Part print with two shaded views. Sizes in mm from the minimum x, y, z corner. Round coordinates to 2 decimals unless told otherwise and drop trailing zeros. Loops run counter-clockwise (first coordinate to the right, second up) from the corner with the lowest first, then second, coordinate; pieces in that order, holes last. Notation, with made-up numbers: (-40, 76.25) - (-4, 76.25) arc R31 cw to (-4, 107.25) - close; hole circle Ø10 at (-20.5, 75). An arc over 180 degrees is marked (long way). Put each result on its own line as item: value. Start each with the question number.
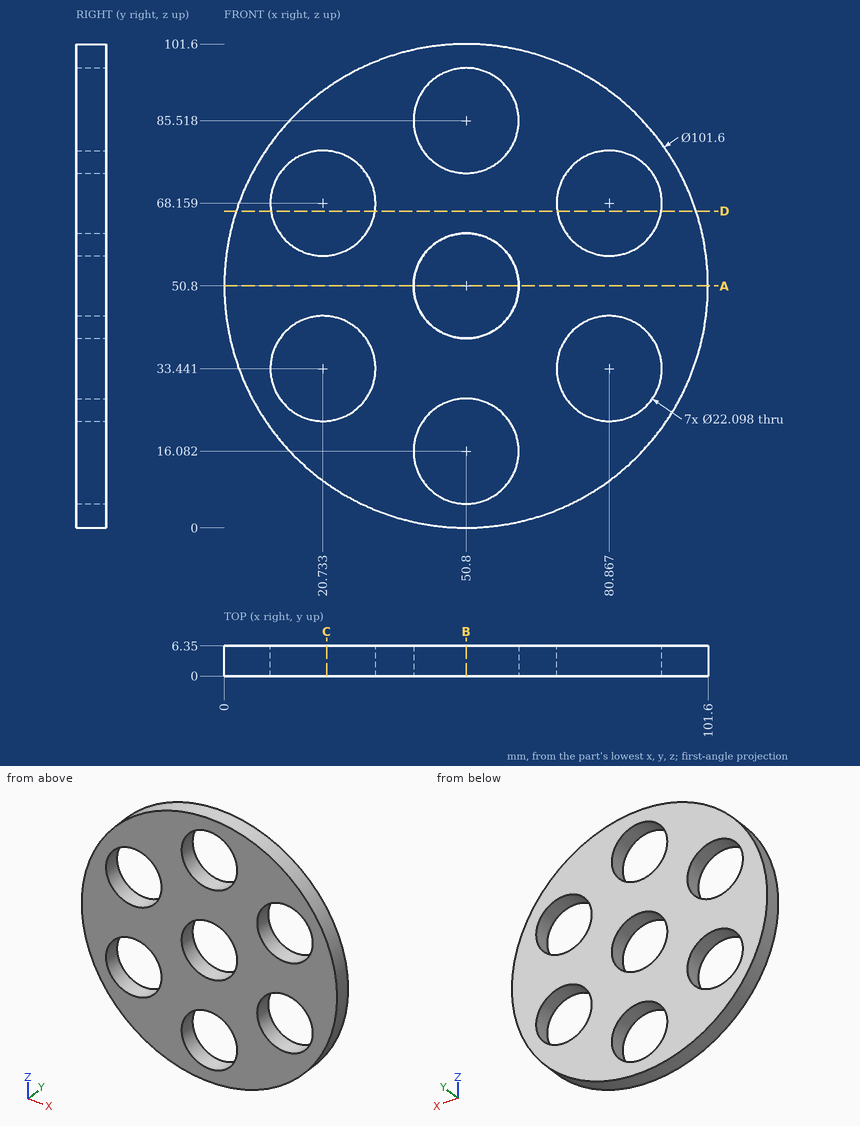
1) Slice it at A-A, the plane z = 50.8. Write the cut outline in (x, y), and give its area (3 significant figures).
2) Slice it at D-D, the plane z = 66.5. Write the cut outline in (x, y).
3) Slice it at C-C, the plane x = 21.5. Write the cut outline in (y, z), and give its area (3 significant figures).
4) Slice it at B-B, the plane x = 50.8. Write the cut outline in (y, z), and give its area (3 significant figures).
5) Drill centre lines: line 1 (Z direction, x = 50, y = 1.25); line 2 (Z direction, x = 50.8, y = 4.25); line 3 (Z direction, x = 88.5, y = 5.5). Where is each one in solid material? Low to high. Write a range as [from, to].
6) Drop flat-ended pins along their axis: pin 1 Ø1.5 at (y, z) = (5, 68.5) entering from +X; pin 2 Ø1.5 at (x, y) = (21.5, 4.5) entering from +Z. Give the stop position or say it passes through.
Taken from the geometry:
1. outline: (0, 0) - (39.75, 0) - (39.75, 6.35) - (0, 6.35) - close; (61.85, 0) - (101.6, 0) - (101.6, 6.35) - (61.85, 6.35) - close
1. area: 505 mm2
2. outline: (2.49, 0) - (9.81, 0) - (9.81, 6.35) - (2.49, 6.35) - close; (31.66, 0) - (69.94, 0) - (69.94, 6.35) - (31.66, 6.35) - close; (91.79, 0) - (99.11, 0) - (99.11, 6.35) - (91.79, 6.35) - close
3. outline: (0, 9.3) - (6.35, 9.3) - (6.35, 22.42) - (0, 22.42) - close; (0, 44.46) - (6.35, 44.46) - (6.35, 57.14) - (0, 57.14) - close; (0, 79.18) - (6.35, 79.18) - (6.35, 92.3) - (0, 92.3) - close
3. area: 247 mm2
4. outline: (0, 0) - (6.35, 0) - (6.35, 5.03) - (0, 5.03) - close; (0, 27.13) - (6.35, 27.13) - (6.35, 39.75) - (0, 39.75) - close; (0, 61.85) - (6.35, 61.85) - (6.35, 74.47) - (0, 74.47) - close; (0, 96.57) - (6.35, 96.57) - (6.35, 101.6) - (0, 101.6) - close
4. area: 224 mm2
5. line 1: z = [0.01, 5.06], [27.1, 39.78], [61.82, 74.5], [96.54, 101.59]
5. line 2: z = [0, 5.03], [27.13, 39.75], [61.85, 74.47], [96.57, 101.6]
5. line 3: z = [16.75, 25.45], [41.43, 60.17], [76.15, 84.85]
6. pin 1: stops at x = 98.69
6. pin 2: stops at z = 92.82
